```python
from build123d import *

# Parameters (mm, degrees)
SKETCH1_R           = 1.75
BOSS_EXTRUDE1_DEPTH = 10


with BuildPart() as part:
    # Sketch1 → Boss-Extrude1 (new body)
    with BuildSketch(Plane.XY):
        with BuildLine():
            Line((0.155, 14.63), (-0.155, 14.63))
            ThreePointArc((-0.155, 14.63), (-0.491925829, 13.37649981), (-0.52, 12.078812028))
            ThreePointArc((-0.52, 12.078812028), (-1.515917744, 11.994586003), (-2.50147536, 11.828386239))
            Line((-2.50147536, 11.828386239), (-11.333513235, 28.769367003))
            ThreePointArc((-11.333513235, 28.769367003), (-15.717822608, 30.148798524), (-17.097254129, 25.764489151))
            Line((-17.097254129, 25.764489151), (-8.265216255, 8.823508388))
            ThreePointArc((-8.265216255, 8.823508388), (-10.691447625, -5.644559122), (2.623945165, -11.801822392))
            ThreePointArc((2.623945165, -11.801822392), (2.986929045, -13.048026405), (3.636804127, -14.171611791))
            Line((3.636804127, -14.171611791), (3.936241133, -14.091377887))
            ThreePointArc((3.936241133, -14.091377887), (3.937256771, -12.793386859), (3.628508025, -11.532650585))
            ThreePointArc((3.628508025, -11.532650585), (4.626642697, -11.169703548), (5.589072804, -10.720558064))
            ThreePointArc((5.589072804, -10.720558064), (6.26222964, -11.830351564), (7.180766062, -12.747451657))
            Line((7.180766062, -12.747451657), (7.449233938, -12.592451657))
            ThreePointArc((7.449233938, -12.592451657), (7.11427017, -11.338425735), (6.489739224, -10.200558064))
            ThreePointArc((6.489739224, -10.200558064), (7.359925677, -9.591641884), (8.173314367, -8.90870542))
            ThreePointArc((8.173314367, -8.90870542), (9.110769635, -9.806457814), (10.235370658, -10.45457376))
            Line((10.235370658, -10.45457376), (10.45457376, -10.235370658))
            ThreePointArc((10.45457376, -10.235370658), (9.806457814, -9.110769635), (8.90870542, -8.173314367))
            ThreePointArc((8.90870542, -8.173314367), (9.591641884, -7.359925677), (10.200558064, -6.489739224))
            ThreePointArc((10.200558064, -6.489739224), (11.338425735, -7.11427017), (12.592451657, -7.449233938))
            Line((12.592451657, -7.449233938), (12.747451657, -7.180766062))
            ThreePointArc((12.747451657, -7.180766062), (11.830351564, -6.26222964), (10.720558064, -5.589072804))
            ThreePointArc((10.720558064, -5.589072804), (11.169703548, -4.626642697), (11.532650585, -3.628508025))
            ThreePointArc((11.532650585, -3.628508025), (12.793386859, -3.937256771), (14.091377887, -3.936241133))
            Line((14.091377887, -3.936241133), (14.171611791, -3.636804127))
            ThreePointArc((14.171611791, -3.636804127), (13.048026405, -2.986929045), (11.801822392, -2.623945165))
            ThreePointArc((11.801822392, -2.623945165), (11.986568374, -1.578061664), (12.078812028, -0.52))
            ThreePointArc((12.078812028, -0.52), (13.37649981, -0.491925829), (14.63, -0.155))
            Line((14.63, -0.155), (14.63, 0.155))
            ThreePointArc((14.63, 0.155), (13.37649981, 0.491925829), (12.078812028, 0.52))
            ThreePointArc((12.078812028, 0.52), (11.986568374, 1.578061664), (11.801822392, 2.623945165))
            ThreePointArc((11.801822392, 2.623945165), (13.048026405, 2.986929045), (14.171611791, 3.636804127))
            Line((14.171611791, 3.636804127), (14.091377887, 3.936241133))
            ThreePointArc((14.091377887, 3.936241133), (12.793386859, 3.937256771), (11.532650585, 3.628508025))
            ThreePointArc((11.532650585, 3.628508025), (11.169703548, 4.626642697), (10.720558064, 5.589072804))
            ThreePointArc((10.720558064, 5.589072804), (11.830351564, 6.26222964), (12.747451657, 7.180766062))
            Line((12.747451657, 7.180766062), (12.592451657, 7.449233938))
            ThreePointArc((12.592451657, 7.449233938), (11.338425735, 7.11427017), (10.200558064, 6.489739224))
            ThreePointArc((10.200558064, 6.489739224), (9.591641884, 7.359925677), (8.90870542, 8.173314367))
            ThreePointArc((8.90870542, 8.173314367), (9.806457814, 9.110769635), (10.45457376, 10.235370658))
            Line((10.45457376, 10.235370658), (10.235370658, 10.45457376))
            ThreePointArc((10.235370658, 10.45457376), (9.110769635, 9.806457814), (8.173314367, 8.90870542))
            ThreePointArc((8.173314367, 8.90870542), (7.359925677, 9.591641884), (6.489739224, 10.200558064))
            ThreePointArc((6.489739224, 10.200558064), (7.11427017, 11.338425735), (7.449233938, 12.592451657))
            Line((7.449233938, 12.592451657), (7.180766062, 12.747451657))
            ThreePointArc((7.180766062, 12.747451657), (6.26222964, 11.830351564), (5.589072804, 10.720558064))
            ThreePointArc((5.589072804, 10.720558064), (4.626642697, 11.169703548), (3.628508025, 11.532650585))
            ThreePointArc((3.628508025, 11.532650585), (3.937256771, 12.793386859), (3.936241133, 14.091377887))
            Line((3.936241133, 14.091377887), (3.636804127, 14.171611791))
            ThreePointArc((3.636804127, 14.171611791), (2.986929045, 13.048026405), (2.623945165, 11.801822392))
            ThreePointArc((2.623945165, 11.801822392), (1.578061664, 11.986568374), (0.52, 12.078812028))
            ThreePointArc((0.52, 12.078812028), (0.491925829, 13.37649981), (0.155, 14.63))
        make_face()
        Circle(SKETCH1_R, mode=Mode.SUBTRACT)
        with Locations((-14.215383682, 27.266928077)):
            Circle(SKETCH1_R, mode=Mode.SUBTRACT)
    extrude(amount=BOSS_EXTRUDE1_DEPTH)


solid = part.part
```
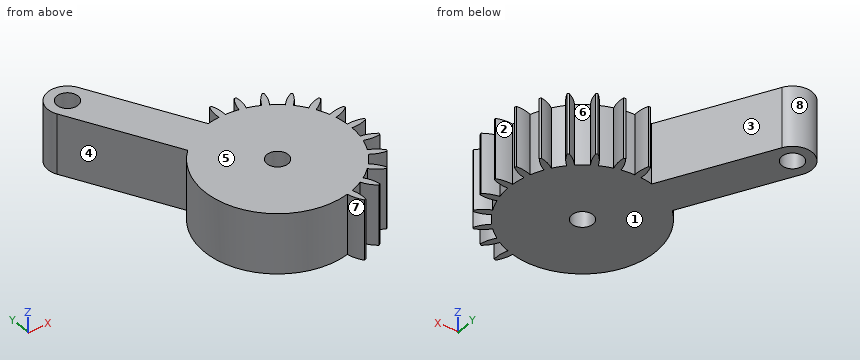
Model file for the job. Use its own axes, mm. Face numbers are marked on the shaded views. A direction names the side the tool comes from. Coordinates: 2 decimals unless noted, no trailing zeros. Write each loop counter-clockwise with the first axis right and the second up, starting at its lowest first coordinate (ties: lowest second). Pieces come first, ordered by that corner, then holes. Notation, with made-up numbers: (89.25, -6) - (103.25, -6) arc R19 cw to (103.25, 31) - close; hole circle Ø7 at (19.25, 61). An arc over 180 degrees is marked (long way). Use a Markdown table: item, result. Add a question column.
Item 1: 3-axis set-ups, long thin cutter, end or side, ignore diameter. For the marked faces 1, 2, 3, 4 and 5: which of +Z, -Z, +X, -X, +Y, -Y reach the whole face in a straight line?
Item 2: Band-saw the part on C-C, the plane z = 7.25. Give the number of separate pieces and of enclosed holes in the cut face, and give its area (3 significant figures).
Item 3: Two-plate mould, pull along Y, no slides. Class the marked faces 6, 7 and 8: pulls with the +Y half, pulls with the -Y half, needs draft (parallel to the pull), parting line crosses it, or undercut.
Item 4: Band-saw the part on B-B, the plane y = 20.5. Write the cut outline in (x, z), and give its area (3 significant figures).
Item 5: Drop flat-ended pins along their axis: pin 1 (4 mm diameter, centred on x = -1.5, z = 3.5, fed in from -Y); pin 2 (1 mm diameter, centred on y = 2.5, z = 1, fed in from +X); pin 3 (2 mm diameter, centred on y = 24.5, z = 3, fed in from +X); pin 4 (12 mm diameter, centred on x = -13, y = -4.5, fed in from -Z). Give the stop position or say it passes through.
Item 6: Band-saw the part on A-A, the plane x = -10. Write the cut outline in (y, z), and give its area (3 significant figures).
Item 7: Drill centre lines: line 1 along Y through (x, z) = (0, 4); line 2 along Y through (x, z) = (7, 8); line 3 along Y through (x, z) = (1.5, 1). Where is each one in solid material? Low to high.
A:
| question | item | result |
|---|---|---|
| 1 | face 1 | -Z, +X, -X, +Y, -Y |
| 1 | face 2 | +Z, -Z |
| 1 | face 3 | +Z, -Z, +Y |
| 1 | face 4 | +Z, -Z, -X |
| 1 | face 5 | +Z, +X, -X, +Y, -Y |
| 2 | separate pieces | 1 |
| 2 | enclosed holes | 2 |
| 2 | area | 606 mm² |
| 3 | face 6 | undercut |
| 3 | face 7 | pulls with the -Y half |
| 3 | face 8 | parting line crosses it |
| 4 | outline | (-14.35, 0) - (-7.02, 0) - (-7.02, 10) - (-14.35, 10) - close |
| 4 | area | 73.3 mm² |
| 5 | pin 1 | stops at y = -12.09 |
| 5 | pin 2 | stops at x = 13.08 |
| 5 | pin 3 | stops at x = -8.59 |
| 5 | pin 4 | stops at z = 0 |
| 6 | outline | (-6.79, 0) - (6.79, 0) - (6.79, 10) - (-6.79, 10) - close; (12.15, 0) - (26.21, 0) - (26.21, 10) - (12.15, 10) - close |
| 6 | area | 276 mm² |
| 7 | line 1 | y = -12.09 to -1.75, 1.75 to 14.63 |
| 7 | line 2 | y = -12.6 to -11.07, -9.86 to 9.86, 11.07 to 12.6 |
| 7 | line 3 | y = -12 to -0.9, 0.9 to 12 |
